from build123d import *

# Parameters (mm, degrees)
F0_R     = 11.0998
F1_DEPTH = 6.9342


with BuildPart() as f1:
    # F0 (on Front) → F1 (new body)
    with BuildSketch(Plane.XZ):
        Polygon((7.125813, 24.379967), (-7.125813, 24.379967), (-12.977696, 11.640459), (-24.379967, 7.125813), (-24.379967, -7.125813), (-12.977696, -11.640459), (-7.125813, -24.379967), (7.125813, -24.379967), (11.467626, -11.640459), (24.379967, -7.125813), (24.379967, 7.125813), (11.467626, 13.130667), align=None)
        Circle(F0_R, mode=Mode.SUBTRACT)
    extrude(amount=-F1_DEPTH)


solid = f1.part
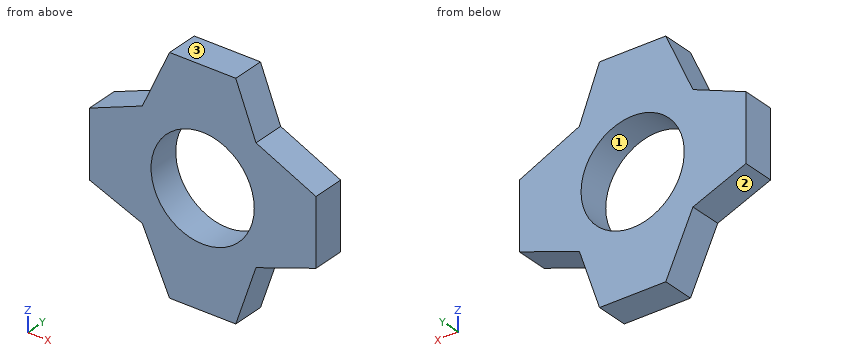
Part model, mm, in its own coordinate system. Face numbers are marked on the shaded views. Coordinates: 2 decimals unless noted, no trailing zeros. Write each loop counter-clockwise with the first axis right and the second up, starting at its lowest first coordinate (ties: lowest second). Pieces come first, ordered by that corner, then holes. Notation, with made-up numbers: (37.25, 74.25) - (68.25, 74.25) arc R26 cw to (68.25, 102.25) - close; hole circle Ø6 at (82, 1.25). An arc over 180 degrees is marked (long way). Put each result on its own line as item: value.
1. Band-saw the part on B-B (x = 0). Write the cut outline in (y, z), then the cut area to 3 significant figures.
Final values:
outline: (0, -24.38) - (6.93, -24.38) - (6.93, -11.1) - (0, -11.1) - close; (0, 11.1) - (6.93, 11.1) - (6.93, 24.38) - (0, 24.38) - close
area: 184 mm²
2. Two-plate mould, pull along Z, no slides. Class the marked faces 1, 2 and 3: +Z half, -Z half, draft (parallel to the pull), parting line (faces both ways), or undercut.
Final values:
face 1: undercut
face 2: -Z half
face 3: +Z half
3. Flat gauge pins, fed straight in: pin 1 Ø2 at (x, y) = (13, 2) entering from +Z; pin 2 Ø1 at (y, z) = (4, 18) entering from +X. Where does each tip first touch, or does it go through?
Final values:
pin 1: stops at z = 12.88
pin 2: stops at x = 9.78
4. Band-saw the part on A-A (y = 1.25). Write the cut outline in (x, z), then the cut area to 3 significant figures.
Final values:
outline: (-24.38, -7.13) - (-12.98, -11.64) - (-7.13, -24.38) - (7.13, -24.38) - (11.47, -11.64) - (24.38, -7.13) - (24.38, 7.13) - (11.47, 13.13) - (7.13, 24.38) - (-7.13, 24.38) - (-12.98, 11.64) - (-24.38, 7.13) - close; hole circle Ø22.2 at (0, 0)
area: 1,140 mm²
5. Band-saw the part on C-C (z = 0). Write the cut outline in (x, y).
Final values:
outline: (-24.38, 0) - (-11.1, 0) - (-11.1, 6.93) - (-24.38, 6.93) - close; (11.1, 0) - (24.38, 0) - (24.38, 6.93) - (11.1, 6.93) - close
6. Probe line 1 along Z through (x, y) = (0.5, 4.25); line 2 along Z through (x, y) = (3.5, 2.5); line 3 along Z through (x, y) = (12.5, 0.75). List the from-to ranges inside material, lowest first. Write a range as [from, to].
Final values:
line 1: z = [-24.38, -11.09], [11.09, 24.38]
line 2: z = [-24.38, -10.53], [10.53, 24.38]
line 3: z = [-11.28, 12.65]
